The drawing under review shows one solid part. Ordinate dimensions are in mm from its lowest x, y, z. Round coordinates to 2 decimals unless told otherwise and drop trailing zeros. Order: outer loops, then holes, each group sorted by start corner. A loop starts at its lowest first (then second) coordinate and runs counter-clockwise, first axis right, second up. Notation, with made-up numbers: (-30.5, 70.25) - (26.5, 70.25) arc R31 cw to (26.5, 95.25) - close; hole circle Ø5 at (73.5, 76). An arc over 180 degrees is marked (long way). One line per question, with ' | ' between items.
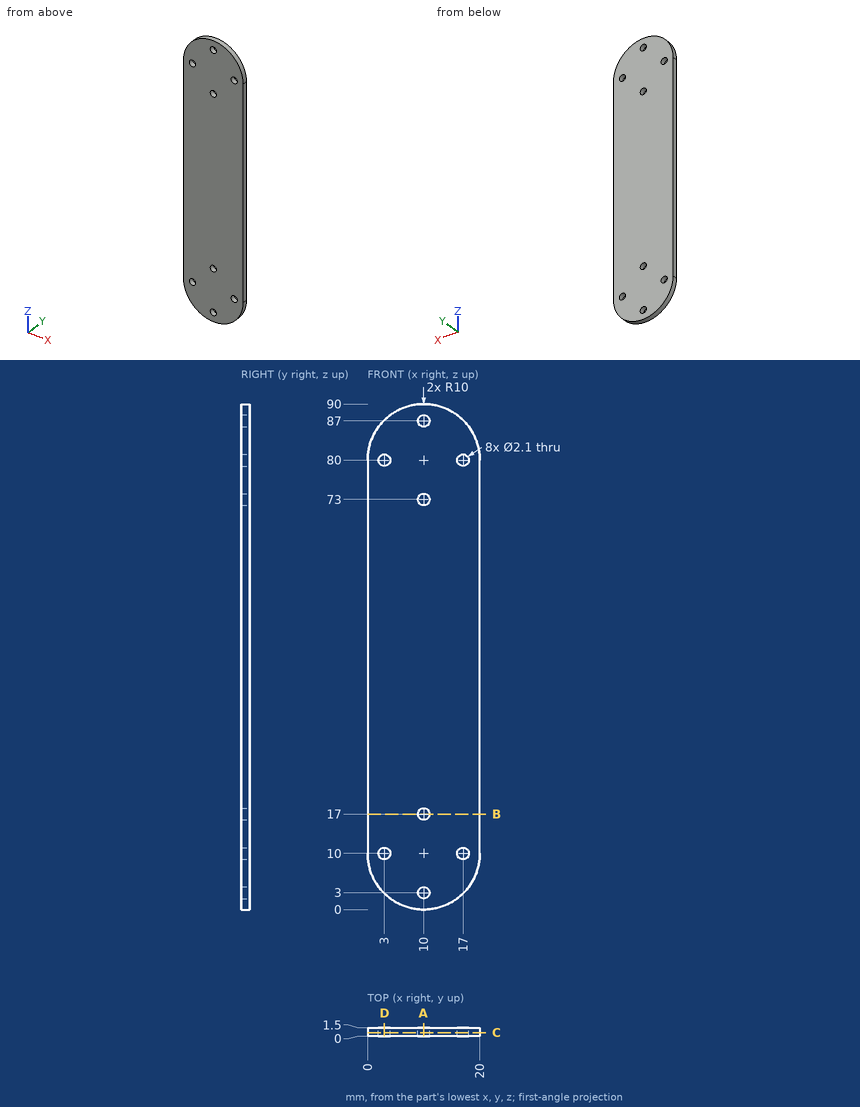
(1) We need section D-D on x = 3. State the section outline as (y, z) points, plus the area to 3 significant figures.
Output values:
outline: (0, 2.86) - (1.5, 2.86) - (1.5, 8.95) - (0, 8.95) - close; (0, 11.05) - (1.5, 11.05) - (1.5, 78.95) - (0, 78.95) - close; (0, 81.05) - (1.5, 81.05) - (1.5, 87.14) - (0, 87.14) - close | area: 120 mm^2
(2) We need section A-A on x = 10. State the section outline as (y, z) points.
Output values:
outline: (0, 0) - (1.5, 0) - (1.5, 1.95) - (0, 1.95) - close; (0, 4.05) - (1.5, 4.05) - (1.5, 15.95) - (0, 15.95) - close; (0, 18.05) - (1.5, 18.05) - (1.5, 71.95) - (0, 71.95) - close; (0, 74.05) - (1.5, 74.05) - (1.5, 85.95) - (0, 85.95) - close; (0, 88.05) - (1.5, 88.05) - (1.5, 90) - (0, 90) - close
(3) Insertion check: pin 1 (2.5 mm diameter, centred on x = 17, z = 10, fed in from -Y). The pin has a flat end and moves straight along its axis. Give the tip position at first contact, or say it passes through.
Output values:
pin 1: y = 0
(4) We need section B-B on z = 17. State the section outline as (x, y) points.
Output values:
outline: (0, 0) - (8.95, 0) - (8.95, 1.5) - (0, 1.5) - close; (11.05, 0) - (20, 0) - (20, 1.5) - (11.05, 1.5) - close
(5) For probe 1 along X at (y, z) = (0.45, 80); probe 2 along Z at (x, y) = (10, 0.6); probe 3 along Z at (x, y) = (17, 0.8), list the stretches that pass through material, from the lowest coordinate up. Write a range as [from, to].
Output values:
probe 1: [0, 1.95], [4.05, 15.95], [18.05, 20] | probe 2: [0, 1.95], [4.05, 15.95], [18.05, 71.95], [74.05, 85.95], [88.05, 90] | probe 3: [2.86, 8.95], [11.05, 78.95], [81.05, 87.14]
(6) We need section C-C on y = 0.6. Give the number of separate pieces and of enclosed holes in the cut face, plus the area to 3 significant figures.
Output values:
separate pieces: 1 | enclosed holes: 8 | area: 1,690 mm^2
